Part model, mm, in its own coordinate system. Face numbers are marked on the shaded views. Round coordinates to 2 decimals unless told otherwise and drop trailing zeros. Loops run counter-clockwise (first coordinate to the right, second up) from the corner with the lowest first, then second, coordinate; pieces in that order, holes last.
1) Drop flat-ended pins along their axis: P1, Ø5, axis at x = 32.5, z = -182, coming from the -Y side; P2, Ø4, axis at x = 32.5, z = -32, coming from the -Y side; P3, Ø1.8, axis at x = 67.5, z = -70, coming from the -Y side; P4, Ø4, axis at y = 37, z = -182.5, coming from the -X side. Give the stop position or say it passes through.
2) Probe line 1 (X direction, y = 33, z = -32); line 2 (Z direction, x = 32.5, y = 32); line 3 (Y direction, x = 1.75, z = -32.5). List the from-to ranges inside material, lowest first.
3) Mould opens along X. For the marked faces 1, 2, 3 and 4 say: +X half, -X half, draft (parallel to the pull), parting line (faces both ways), or undercut.
4) Band-saw the part on A-A, the plane y = 26.5. Write the cut outline in (x, z), then the cut area to 3 significant figures.
5) Band-saw the part on B-B, the plane x = 54. Write the cut outline in (y, z), then the cut area to 3 significant figures.
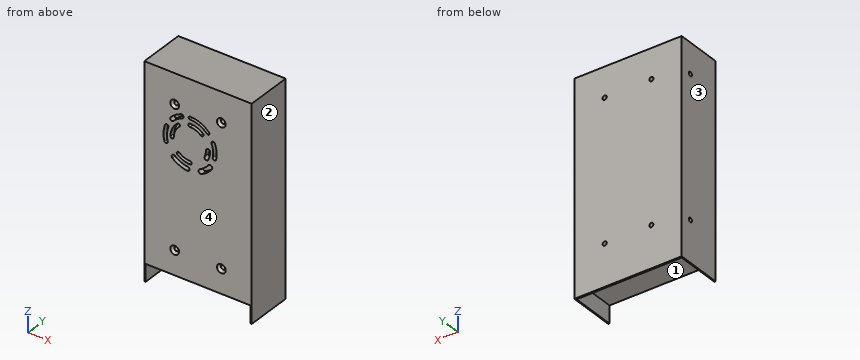
from build123d import *

# Parameters (mm, degrees)
SKETCH3_W                                       = 115
SKETCH3_H                                       = 226.5
BOSS_EXTRUDE1_DEPTH                             = 49.7
CSK_FOR_M4_FLAT_HEAD_MACHINE_SCREW2_D           = 4.5
CSK_FOR_M4_FLAT_HEAD_MACHINE_SCREW2_CSINK_D     = 9.4
CSK_FOR_M4_FLAT_HEAD_MACHINE_SCREW2_CSINK_ANGLE = 90
SKETCH8_W                                       = 112.444388117
SKETCH8_H                                       = 18.583241451
CUT_EXTRUDE1_DEPTH                              = 48
CUT_EXTRUDE2_DEPTH                              = 6
M4_CLEARANCE_HOLE1_D                            = 4.5
M4_CLEARANCE_HOLE1_DEPTH                        = 5
M4_CLEARANCE_HOLE1_TIP                          = 1.351936393


with BuildPart() as part:
    # Sketch3 → Boss-Extrude1 (new body)
    with BuildSketch(Plane(origin=(0, 0, 0), x_dir=(1, 0, 0), z_dir=(0, 1, 0))):
        with Locations((57.5, 113.25)):
            Rectangle(SKETCH3_W, SKETCH3_H)
    extrude(amount=BOSS_EXTRUDE1_DEPTH)

    # CSK for M4 Flat Head Machine Screw2 (through all)
    with Locations(Plane(origin=(0, 0, 0), x_dir=(-1, 0, 0), z_dir=(0, -1, 0))):
        with Locations((-32.5, 32), (-82.5, 32), (-82.5, 182), (-32.5, 182)):
            CounterSinkHole(CSK_FOR_M4_FLAT_HEAD_MACHINE_SCREW2_D / 2, CSK_FOR_M4_FLAT_HEAD_MACHINE_SCREW2_CSINK_D / 2, counter_sink_angle=CSK_FOR_M4_FLAT_HEAD_MACHINE_SCREW2_CSINK_ANGLE)

    # Sketch8 → Cut-Extrude1 (cut)
    with BuildSketch(Plane(origin=(0, 0, 0), x_dir=(-1, 0, 0), z_dir=(0, -1, 0))):
        with Locations((-57.518541752, 217.208379275)):
            Rectangle(SKETCH8_W, SKETCH8_H)
    extrude(amount=-CUT_EXTRUDE1_DEPTH, mode=Mode.SUBTRACT)

    # Sketch9 → Cut-Extrude2 (cut)
    with BuildSketch(Plane(origin=(0, 0, 0), x_dir=(-1, 0, 0), z_dir=(0, -1, 0))):
        with BuildLine():
            ThreePointArc((-35.24160151, 50.698787363), (-29.906155704, 57.837710564), (-28.013949561, 66.546944878))
            ThreePointArc((-28.013949561, 66.546944878), (-29.740661802, 68.27365712), (-31.467374044, 66.546944878))
            ThreePointArc((-31.467374044, 66.546944878), (-33.0482468, 59.270680978), (-37.505827146, 53.306357674))
            ThreePointArc((-37.505827146, 53.306357674), (-37.677499484, 50.870459701), (-35.24160151, 50.698787363))
        make_face()
        with BuildLine():
            ThreePointArc((-62.815145497, 50.64033664), (-56.375233323, 46.812564416), (-49.002996311, 45.480486923))
            ThreePointArc((-49.002996311, 45.480486923), (-47.198872865, 47.284610369), (-49.002996311, 49.088733815))
            ThreePointArc((-49.002996311, 49.088733815), (-55.112522176, 50.192654089), (-60.449411092, 53.364808398))
            ThreePointArc((-60.449411092, 53.364808398), (-62.994514173, 53.185439721), (-62.815145497, 50.64033664))
        make_face()
        with BuildLine():
            ThreePointArc((-68.572182043, 75.27774008), (-69.961499926, 71.01023305), (-70.43147771, 66.546944878))
            ThreePointArc((-70.43147771, 66.546944878), (-68.26533082, 64.380797988), (-66.09918393, 66.546944878))
            ThreePointArc((-66.09918393, 66.546944878), (-65.724223696, 70.107869732), (-64.615790544, 73.512595409))
            ThreePointArc((-64.615790544, 73.512595409), (-65.711413958, 76.373363494), (-68.572182043, 75.27774008))
        make_face()
        with BuildLine():
            ThreePointArc((-35.258623929, 82.375498714), (-41.66693518, 86.184487896), (-49.002996311, 87.510028828))
            ThreePointArc((-49.002996311, 87.510028828), (-50.703745752, 85.809279387), (-49.002996311, 84.108529946))
            ThreePointArc((-49.002996311, 84.108529946), (-42.857294566, 82.998073111), (-37.488804727, 79.807135761))
            ThreePointArc((-37.488804727, 79.807135761), (-35.089532852, 79.976226838), (-35.258623929, 82.375498714))
        make_face()
        with BuildLine():
            ThreePointArc((-69.40308911, 47.094937136), (-60.098890521, 40.635064917), (-49.002996311, 38.359281062))
            ThreePointArc((-49.002996311, 38.359281062), (-47.430907963, 39.93136941), (-49.002996311, 41.503457758))
            ThreePointArc((-49.002996311, 41.503457758), (-58.861205404, 43.525390616), (-67.12757253, 49.264700116))
            ThreePointArc((-67.12757253, 49.264700116), (-69.35021231, 49.317576916), (-69.40308911, 47.094937136))
        make_face()
        with BuildLine():
            ThreePointArc((-76.955702254, 72.084205228), (-77.381483247, 63.963052285), (-75.495983574, 56.052344001))
            ThreePointArc((-75.495983574, 56.052344001), (-73.055355825, 54.99668972), (-71.999701544, 57.437317469))
            ThreePointArc((-71.999701544, 57.437317469), (-73.636371647, 64.304048834), (-73.266781011, 71.353452457))
            ThreePointArc((-73.266781011, 71.353452457), (-74.745865247, 73.563289464), (-76.955702254, 72.084205228))
        make_face()
        with BuildLine():
            ThreePointArc((-61.479475854, 92.737765271), (-67.474162168, 88.917408587), (-72.359830302, 83.7539179))
            ThreePointArc((-72.359830302, 83.7539179), (-71.852094521, 80.404948498), (-68.503125119, 80.912684278))
            ThreePointArc((-68.503125119, 80.912684278), (-64.424183685, 85.223573911), (-59.419346329, 88.41310925))
            ThreePointArc((-59.419346329, 88.41310925), (-58.287083081, 91.605502023), (-61.479475854, 92.737765271))
        make_face()
        with BuildLine():
            ThreePointArc((-30.044644277, 88.193682414), (-37.532685074, 92.936949007), (-46.109148954, 95.176056029))
            ThreePointArc((-46.109148954, 95.176056029), (-48.474789772, 93.244752833), (-46.543486577, 90.879112015))
            ThreePointArc((-46.543486577, 90.879112015), (-39.254264376, 88.976072623), (-32.890103811, 84.944723032))
            ThreePointArc((-32.890103811, 84.944723032), (-29.842894353, 85.146472956), (-30.044644277, 88.193682414))
        make_face()
        with BuildLine():
            ThreePointArc((-22.242703071, 56.799039322), (-20.547999949, 65.343558372), (-21.515231892, 74.000652968))
            ThreePointArc((-21.515231892, 74.000652968), (-23.803146789, 75.312452747), (-25.114946569, 73.02453785))
            ThreePointArc((-25.114946569, 73.02453785), (-24.274380402, 65.501150237), (-25.747150317, 58.075595617))
            ThreePointArc((-25.747150317, 58.075595617), (-24.633204841, 55.685093846), (-22.242703071, 56.799039322))
        make_face()
        with BuildLine():
            ThreePointArc((-39.301431481, 39.586636452), (-33.365347236, 42.53772744), (-28.266328256, 46.774004062))
            ThreePointArc((-28.266328256, 46.774004062), (-28.334847238, 49.654152172), (-31.214995349, 49.58563319))
            ThreePointArc((-31.214995349, 49.58563319), (-35.588955249, 45.951737309), (-40.680953248, 43.420279064))
            ThreePointArc((-40.680953248, 43.420279064), (-41.90801367, 40.813696874), (-39.301431481, 39.586636452))
        make_face()
    extrude(amount=-CUT_EXTRUDE2_DEPTH, mode=Mode.SUBTRACT)

    # M4 Clearance Hole1
    with Locations(Plane.ZY):
        with Locations((-32.5, 37), (-182.5, 37)):
            Hole(M4_CLEARANCE_HOLE1_D / 2, depth=M4_CLEARANCE_HOLE1_DEPTH)
            with Locations((0, 0, -(M4_CLEARANCE_HOLE1_DEPTH + M4_CLEARANCE_HOLE1_TIP / 2))):  # 118° drill point
                Cone(0, M4_CLEARANCE_HOLE1_D / 2, M4_CLEARANCE_HOLE1_TIP, mode=Mode.SUBTRACT)


solid = part.part
Reported:
1. P1: stops at y = 2.2
1. P2: passes through
1. P3: stops at y = 6
1. P4: stops at x = 5.15
2. line 1: x = 0 to 30.25, 34.75 to 80.25, 84.75 to 115
2. line 2: z = -207.92 to -184.25, -179.75 to -34.25, -29.75 to 0
2. line 3: y = 0 to 34.75, 39.25 to 49.7
3. face 1: undercut
3. face 2: +X half
3. face 3: -X half
3. face 4: draft
4. outline: (0, -226.5) - (1.3, -226.5) - (1.3, -207.92) - (113.74, -207.92) - (113.74, -226.5) - (115, -226.5) - (115, 0) - (0, 0) - close; hole circle Ø4.5 at (32.5, -182); hole circle Ø4.5 at (32.5, -32); hole circle Ø4.5 at (82.5, -182); hole circle Ø4.5 at (82.5, -32)
4. area: 23,900 mm2
5. outline: (0, -207.92) - (48, -207.92) - (48, -226.5) - (49.7, -226.5) - (49.7, 0) - (0, 0) - (0, -38.81) - (6, -38.81) - (6, -42.01) - (0, -42.01) - (0, -46.08) - (6, -46.08) - (6, -49.82) - (0, -49.82) - close
5. area: 10,300 mm2
